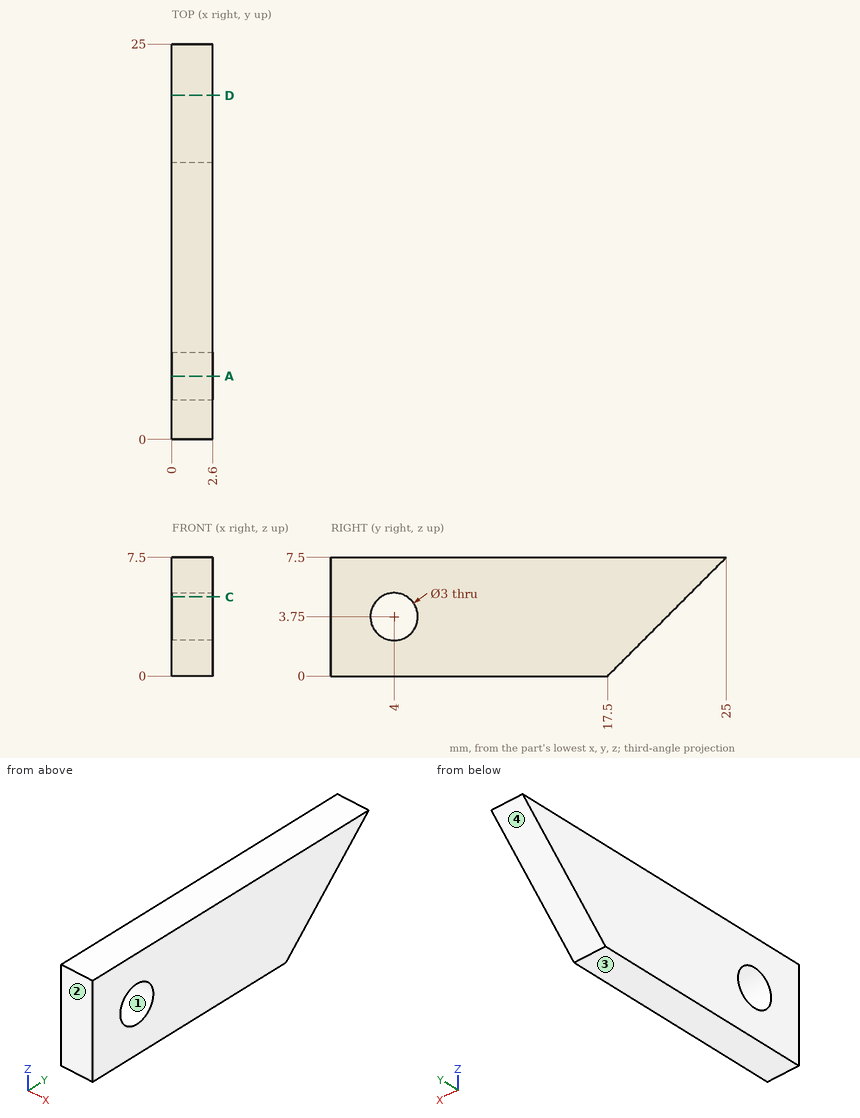
Geometry check sheet. Reference: drawing and pictorial views, mm from the part's lowest x, y, z. Give positions to 0.01 mm unless a question says otherwise; leave off trailing zeros. Order: outer loops, then holes, each group sorted by start corner. A loop starts at its lowest first (then second) coordinate and runs counter-clockwise, first axis right, second up. Notation, with made-up numbers: (19, 88.25) -> (76, 88.25) arc R21 cw to (76, 103.25) -> close; hole circle Ø5 at (-22.5, 12.25). An arc over 180 degrees is marked (long way). Use CSV: the item, a comma, the result in double quotes. Start each with the question number.
1) Sectioned sample at C-C, the plane z = 5. Record the boundary of the cut face in (x, y).
2) Material ranges on line 1 (Y direction, x = 1.15, z = 3.75); line 2 (Z direction, x = 1.5, y = 22.75); line 3 (Y direction, x = 0.5, z = 3.5), recorded low to high. Write a range as from..to.
3) Sectioned sample at A-A, the plane y = 4. Record the boundary of the cut face in (x, z).
4) Go/stop test with a flat-tipped pin: P1, Ø1, axis at x = 1, z = 6.5, coming from the +Y side. Record where the tip stops, or that it passes through.
5) Sectioned sample at D-D, the plane y = 21.75. Record the boundary of the cut face in (x, z).
6) Mould release check, pull along Y, two halves, no side actions. Record for the marked faces 1, 2, 3 and 4: released by +Y, released by -Y, zero draft, split by the parting line, or undercut.
Recorded:
1,outline,"(0, 0) -> (2.6, 0) -> (2.6, 3.17) -> (0, 3.17) -> close; (0, 4.83) -> (2.6, 4.83) -> (2.6, 22.5) -> (0, 22.5) -> close"
2,line 1,"0..2.5, 5.5..21.25"
2,line 2,"5.25..7.5"
2,line 3,"0..2.52, 5.48..21"
3,outline,"(0, 0) -> (2.6, 0) -> (2.6, 2.25) -> (0, 2.25) -> close; (0, 5.25) -> (2.6, 5.25) -> (2.6, 7.5) -> (0, 7.5) -> close"
4,P1,"y = 24.5"
5,outline,"(0, 4.25) -> (2.6, 4.25) -> (2.6, 7.5) -> (0, 7.5) -> close"
6,face 1,"undercut"
6,face 2,"released by -Y"
6,face 3,"zero draft"
6,face 4,"released by +Y"
